Part model, mm, in its own coordinate system. A direction names the side the tool comes from. Give positions to 0.01 mm unless a question says otherwise; leave off trailing zeros. Order: outer loops, then holes, each group sorted by start corner. A loop starts at its lowest first (then second) coordinate and runs counter-clockwise, first axis right, second up. Notation, with made-up numbers: (-38, 59.5) - (-3, 59.5) arc R17 cw to (-3, 83.5) - close; hole circle Ø8 at (20.5, -38). An arc over 180 degrees is marked (long way). One line per item, written item: value.
```python
from build123d import *
from build123d.topology import SkipClean

# Parameters (mm, degrees)
SKETCH_1_R      = 1.5
EXTRUDE_1_DEPTH = 3
SKETCH_2_R      = 1.5
EXTRUDE_2_DEPTH = 7
CHAMFER_1_SIZE  = 1.5
FILLET_1_R      = 0.7
FILLET_2_R      = 0.5
SKETCH_3_R      = 3
SKETCH_3_R_2    = 1.5
EXTRUDE_3_DEPTH = 2.22
FILLET_3_R      = 0.5


with BuildPart() as part:
    # 草图1 → 凸台-拉伸1 (new body)
    with BuildSketch(Plane.XY):
        with BuildLine():
            Line((-14.399999999, 4.45), (-14.399999999, -12.55))
            ThreePointArc((-14.399999999, -12.55), (-17.899999999, -16.05), (-21.399999999, -12.55))
            Line((-21.399999999, -12.55), (-21.399999999, 4.45))
            ThreePointArc((-21.399999999, 4.45), (-17.899999999, 7.95), (-14.399999999, 4.45))
        make_face()
        with Locations((-17.899999999, 4.45)):
            Circle(SKETCH_1_R, mode=Mode.SUBTRACT)
        with Locations((-17.899999999, -12.55)):
            Circle(SKETCH_1_R, mode=Mode.SUBTRACT)
    extrude(amount=EXTRUDE_1_DEPTH)

    # 草图2 → 凸台-拉伸2 (add)
    with BuildSketch(Plane(origin=(-14.399999999, 0, 0), x_dir=(0, 0, -1), z_dir=(1, 0, 0))):
        with BuildLine():
            Line((-6.132588308, 0.199416458), (-3, 0.199416458))
            Line((-3, 0.199416458), (-3, -6.800583542))
            Line((-3, -6.800583542), (-6.132588308, -6.800583542))
            ThreePointArc((-6.132588308, -6.800583542), (-9.632588308, -3.300583542), (-6.132588308, 0.199416458))
        make_face()
        with Locations(Location((-6.132588308, -3.300583542, 0), (0, 0, 90))):
            Circle(SKETCH_2_R, mode=Mode.SUBTRACT)
    extrude(amount=-EXTRUDE_2_DEPTH)

    # 倒角1
    chamfer_1_edges = [part.edges().sort_by_distance(p)[0] for p in [
        (-14.399999999, -4.800583542, 6.132588308),
    ]]
    chamfer(chamfer_1_edges, length=CHAMFER_1_SIZE)

    # 圆角1
    fillet_1_edges = [part.edges().sort_by_distance(p)[0] for p in [
        (-17.899999999, -6.800583542, 3),
        (-17.899999999, 0.199416458, 3),
    ]]
    fillet(fillet_1_edges, radius=FILLET_1_R)

    # 圆角2
    fillet_2_edges = [part.edges().sort_by_distance(p)[0] for p in [
        (-17.899999999, -16.05, 3),
        (-14.399999999, -10.025291771, 3),
        (-14.399999999, -3.300583542, 9.632588308),
        (-14.399999999, -6.800583542, 4.916294154),
        (-21.399999999, -3.300583542, 9.632588308),
        (-21.399999999, 0.199416458, 4.916294154),
        (-14.399999999, 2.674708229, 3),
        (-14.399999999, 0.199416458, 4.916294154),
        (-21.399999999, -6.800583542, 4.916294154),
        (-21.399999999, -10.025291771, 3),
        (-14.399999999, 0.404441711, 3.205025253),
        (-21.399999999, 0.404441711, 3.205025253),
        (-14.399999999, -7.005608796, 3.205025253),
        (-21.399999999, -7.005608796, 3.205025253),
        (-17.899999999, 7.95, 3),
        (-21.399999999, 2.674708229, 3),
    ]]
    fillet(fillet_2_edges, radius=FILLET_2_R - 0.0001)  # a hair under: the kernel refuses the full size

    # 草图3 → 凸台-拉伸3 (add)
    with SkipClean():  # the faces are left unmerged after this step: merging them gives an invalid solid
        with BuildSketch(Plane.ZY.offset(21.399999999)):
            with Locations(Location((6.132588308, -3.300583542, 0), (0, 0, 270))):
                Circle(SKETCH_3_R)
            with Locations(Location((6.132588308, -3.300583542, 0), (0, 0, 270))):
                Circle(SKETCH_3_R_2, mode=Mode.SUBTRACT)
        extrude(amount=EXTRUDE_3_DEPTH)
    add(part.part.scale(1), mode=Mode.REPLACE)  # the faces are merged on a copy

    # 圆角3
    fillet_3_edges = [part.edges().sort_by_distance(p)[0] for p in [
        (-21.399999999, -0.300583542, 6.132588308),
        (-21.399999999, -0.300583542, 6.132588308),
    ]]
    fillet(fillet_3_edges, radius=FILLET_3_R)


solid = part.part
```
1) Cut at C-C, the plane z = 0.5. Give the cut face in (x, y), then the cut area to 3 significant figures.
Outcome:
outline: (-21.4, -12.55) arc R3.5 ccw to (-14.4, -12.55) - (-14.4, 4.45) arc R3.5 ccw to (-21.4, 4.45) - close; hole circle Ø3 at (-17.9, -12.55); hole circle Ø3 at (-17.9, 4.45)
area: 143 mm^2
2) Drill centre lines: line 1 along Y through (x, z) = (-17.9, 2.1); line 2 along Y through (x, z) = (-18.5, 1.5); line 3 along Z through (x, y) = (-14.75, -1.75). Where is each one in solid material? Low to high. Write a range as from..to.
Outcome:
line 1: y = -16.05..-14.05, -11.05..2.95, 5.95..7.95
line 2: y = -16..-13.92, -11.18..3.08, 5.82..7.9
line 3: z = 0..3.98, 8.28..9.24
3) Cut at A-A, the plane x = -17.9. Give the number of separate pieces and of enclosed holes in the cut face, then the cut area to 3 significant figures.
Outcome:
separate pieces: 3
enclosed holes: 1
area: 88.2 mm^2
4) Cut at B-B, the plane y = -8. Give the cut face in (x, z).
Outcome:
outline: (-21.4, 0) - (-14.4, 0) - (-14.4, 2.5) arc R0.5 ccw to (-14.9, 3) - (-20.9, 3) arc R0.5 ccw to (-21.4, 2.5) - close
5) Which spindle directions (+Z, -Z, +X, -X, +Y, -Y) get a long thin tool onto all of the face, cutting with end or side? Do faces 1 (the flat face through (-18, -6.801, 5)), 2 (the flat face through (-18, 0.199, 5)), 3 (the cylindrical face through (-22.68, -2.91, 9.107)), 4 (the flat face through (-23.62, -4, 8)). Say none if no direction does.
Outcome:
face 1: +Z, +X, -X, -Y
face 2: +Z, +X, -X, +Y
face 3: -X
face 4: +Z, -Z, -X, +Y, -Y
6) Cut at D-D, the plane x = -23. Give the cut face in (y, z).
Outcome:
outline: circle Ø6 at (-3.3, 6.13); hole circle Ø3 at (-3.3, 6.13)
7) Pin check, flat tips, straight feed: pin 1 (5 mm diameter, centred on x = -17, y = 3, fed in from +Z); pin 2 (1.8 mm diameter, centred on x = -17.9, y = -12.55, fed in from +Z); pin 3 (4 mm diameter, centred on x = -20.5, z = 8.5, fed in from +Y); pin 4 (3 mm diameter, centred on x = -19, y = -11.5, fed in from +Z). Stop position of each tip, or through.
Outcome:
pin 1: stops at z = 3.13
pin 2: passes through
pin 3: stops at y = 0.18
pin 4: stops at z = 3
